Input: part model. Units: mm. Frame: model coordinates. Face numbers are marked on the shaded views. A direction names the side the tool comes from. Coordinates: 2 decimals unless noted, no trailing zeros. Write each loop counter-clockwise with the first axis right and the second up, starting at its lowest first coordinate (ties: lowest second). Pieces come first, ordered by that corner, then holes. Notation, with made-up numbers: (73, 11) -> (106, 11) arc R15 ccw to (106, 39) -> close; hole circle Ø10 at (-12, -34.75). An arc over 180 degrees is marked (long way). One line per question, with ' | ' between items. Start each with the question number.
```python
from build123d import *

# Parameters (mm, degrees)
F0_W     = 15
F0_H     = 15
F0_R     = 5
F1_DEPTH = 5
F3_DEPTH = 5
F5_DEPTH = 5
F7_DEPTH = 2.5


with BuildPart() as f1:
    # F0 (on Top) → F1 (new body, symmetric)
    with BuildSketch(Plane.XY):
        Rectangle(F0_W, F0_H)
        Circle(F0_R, mode=Mode.SUBTRACT)
    extrude(amount=F1_DEPTH, both=True)

    # F2 (on Top) → F3 (join, symmetric)
    with BuildSketch(Plane.XY):
        with BuildLine():
            Line((13.7621368783, 2.8581836929), (7.5, 7.5))
            Line((7.5, 7.5), (7.5, -7.5))
            Line((7.5, -7.5), (13.7621368783, -2.8581836929))
            Line((13.7621368783, -2.8581836929), (13.7621368783, -2.6422807153))
            ThreePointArc((13.7621368783, -2.6422807153), (10.25, 0), (13.7621368783, 2.6422807153))
            Line((13.7621368783, 2.6422807153), (13.7621368783, 2.8581836929))
        make_face()
    extrude(amount=F3_DEPTH, both=True)

    # F4 (on Top) → F5 (join, symmetric)
    with BuildSketch(Plane.XY):
        with BuildLine():
            Line((-7.5, 7.5), (-11.2602819583, 2.1297608165))
            ThreePointArc((-11.2602819583, 2.1297608165), (-15.75, 0), (-11.2602819583, -2.1297608165))
            Line((-11.2602819583, -2.1297608165), (-7.5, -7.5))
            Line((-7.5, -7.5), (-7.5, 7.5))
        make_face()
    extrude(amount=F5_DEPTH, both=True)

    # F6 (on Top) → F7 (cut, symmetric)
    with BuildSketch(Plane.XY):
        with BuildLine():
            Line((-7.5, -2.1297608165), (-7.5, 2.1297608165))
            Line((-7.5, 2.1297608165), (-7.5, 7.5))
            Line((-7.5, 7.5), (-11.2602819583, 7.5))
            Line((-11.2602819583, 7.5), (-11.2602819583, 2.1297608165))
            ThreePointArc((-11.2602819583, 2.1297608165), (-10.25, 0), (-11.2602819583, -2.1297608165))
            Line((-11.2602819583, -2.1297608165), (-11.2602819583, -7.5))
            Line((-11.2602819583, -7.5), (-7.5, -7.5))
            Line((-7.5, -7.5), (-7.5, -2.1297608165))
        make_face()
        Polygon((7.5, 7.5), (7.5, 2.8581836929), (7.5, -2.8581836929), (7.5, -7.5), (13.7621368783, -7.5), (13.7621368783, -2.8581836929), (13.7621368783, 2.8581836929), (13.7621368783, 7.5), align=None)
    extrude(amount=F7_DEPTH, both=True, mode=Mode.SUBTRACT)


solid = f1.part
```
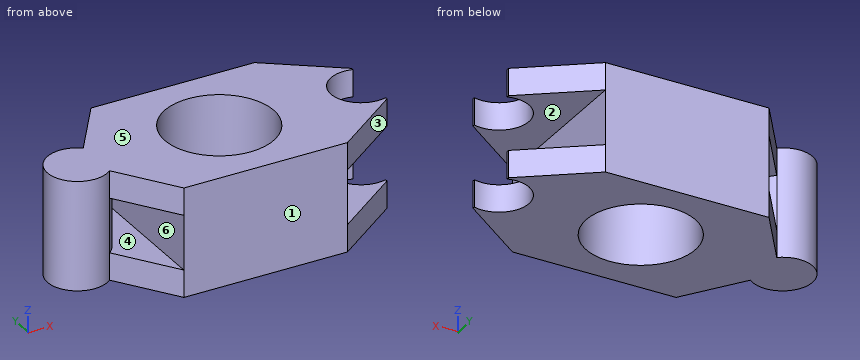
1) Access query for the marked faces 1 and 2. Directions: +Z, -Z, +X, -X, +Y, -Y. A direction counts if a zero-diameter tool reaches every point of the face in a straight line with its end or side. Return the directions, or none.
2) Section C-C, the plane z = 2. Return loops of the section in (x, y).
3) Ray query, line 1 (Z direction, x = 10, y = -5); line 2 (Y direction, x = 0, z = -2.25); line 3 (X direction, y = -1.5, z = 0). Return the intervals inside material, ascending.
4) Section D-D, the plane z = 3.25. Return loops of the section in (x, y).
5) Section A-A, the plane y = 0. Return loops of the section in (x, z), then the cut area to 4 significant figures.
6) First-contact query: P1, Ø2, axis at y = 6, z = 3.5, coming from the -X side; P2, Ø3, axis at y = 2.5, z = -2, coming from the -X side; P3, Ø1.5, axis at y = -2, z = -1, coming from the -X side. Flat tips, straight axial feed; report the tip coordinate or a pass-through.
7) Section B-B, the plane x = 0. Return loops of the section in (y, z), then the cut area to 3 significant figures.
8) Pull-direction query (Z, two-part tool) for the marked faces 3, 4, 5 and 6; classes: released by +Z, released by -Z, zero draft, split by the parting line, or undercut.
Answer block:
1) face 1: +Z, -Z, +X, -X, -Y | face 2: +X, +Y, -Y
2) outline: circle Ø5.5 at (-13, 0); (-7.5, -7.5) -> (7.5, -7.5) -> (7.5, 7.5) -> (-7.5, 7.5) -> close; hole circle Ø10 at (0, 0)
3) line 1: z = -5 to -2.5, 2.5 to 5 | line 2: y = -7.5 to -5, 5 to 7.5 | line 3: x = -15.3 to -10.7, -7.5 to -4.77, 4.77 to 7.5
4) outline: (-11.26, -2.13) -> (-7.5, -7.5) -> (7.5, -7.5) -> (13.76, -2.86) -> (13.76, -2.64) arc R2.75 cw (long way) to (13.76, 2.64) -> (13.76, 2.86) -> (7.5, 7.5) -> (-7.5, 7.5) -> (-11.26, 2.13) arc R2.75 ccw (long way) to start; hole circle Ø10 at (0, 0)
5) outline: (-15.75, -5) -> (-5, -5) -> (-5, 5) -> (-15.75, 5) -> close; (5, -5) -> (10.25, -5) -> (10.25, -2.5) -> (7.5, -2.5) -> (7.5, 2.5) -> (10.25, 2.5) -> (10.25, 5) -> (5, 5) -> close; hole (-10.25, -2.5) -> (-7.5, -2.5) -> (-7.5, 2.5) -> (-10.25, 2.5) -> close | area: 132.5 mm2
6) P1: stops at x = -9.25 | P2: stops at x = -15.56 | P3: stops at x = -15.45
7) outline: (-7.5, -5) -> (-5, -5) -> (-5, 5) -> (-7.5, 5) -> close; (5, -5) -> (7.5, -5) -> (7.5, 5) -> (5, 5) -> close | area: 50.0 mm2
8) face 3: zero draft | face 4: undercut | face 5: released by +Z | face 6: undercut
